Answer from the drawing. Dimensions are ordinates in mm from the lowest x, y and z of the part. A direction names the side the tool comes from. Give positions to 0.01 mm unless a question says otherwise; leave off trailing zeros. Order: outer loops, then holes, each group sorted by start corner. A loop starts at its lowest first (then second) coordinate and runs counter-clockwise, first axis right, second up. Notation, with made-up numbers: (-39, 30.5) - (-3, 30.5) arc R13 cw to (-3, 51.5) - close; hole circle Ø9 at (20.5, -10). An arc over 180 degrees is marked (long way). Use a Markdown table: item, result. Add a question column.
1) Find section D-D, the plane x = 18.25. Determine the outline of the cut face in (y, z).
2) Find section A-A, the plane x = 4. Determine the outline of the cut face in (y, z).
3) Find section C-C, the plane y = 3.5. Determine the outline of the cut face in (x, z), plus the area to 3 significant figures.
4) Find section B-B, the plane z = 10.5. Determine the outline of the cut face in (x, y).
5) Flat-ended cylindrical pins translate along their axes: pin 1 (6 mm diameter, centred on x = 12, z = 7.5, fed in from +Y); pin 2 (1.5 mm diameter, centred on x = 4, y = 4, fed in from +Z); pin 3 (1.5 mm diameter, centred on x = 4, z = 6, fed in from +Y). Find the tip coordinate at first contact, or state that the pin passes through.
6) For the marked faces 1 and 2, determine the directions among +Z, -Z, +X, -X, +Y, -Y from which every point of the face is accessible in a straight line to the end or side of a thin tool.
7) Straight lines are drawn through the part: line 1 (X direction, y = 0.5, z = 10.5); line 2 (Y direction, x = 2.15, z = 3); line 3 (X direction, y = 1.2, z = 4.5). For each, find the intervals that lie inside material, in ascending order.
8) The mould has two halves that part along X. Classify the marked faces 3, 4, 5 and 6: released by +X, released by -X, zero draft, split by the parting line, or undercut.
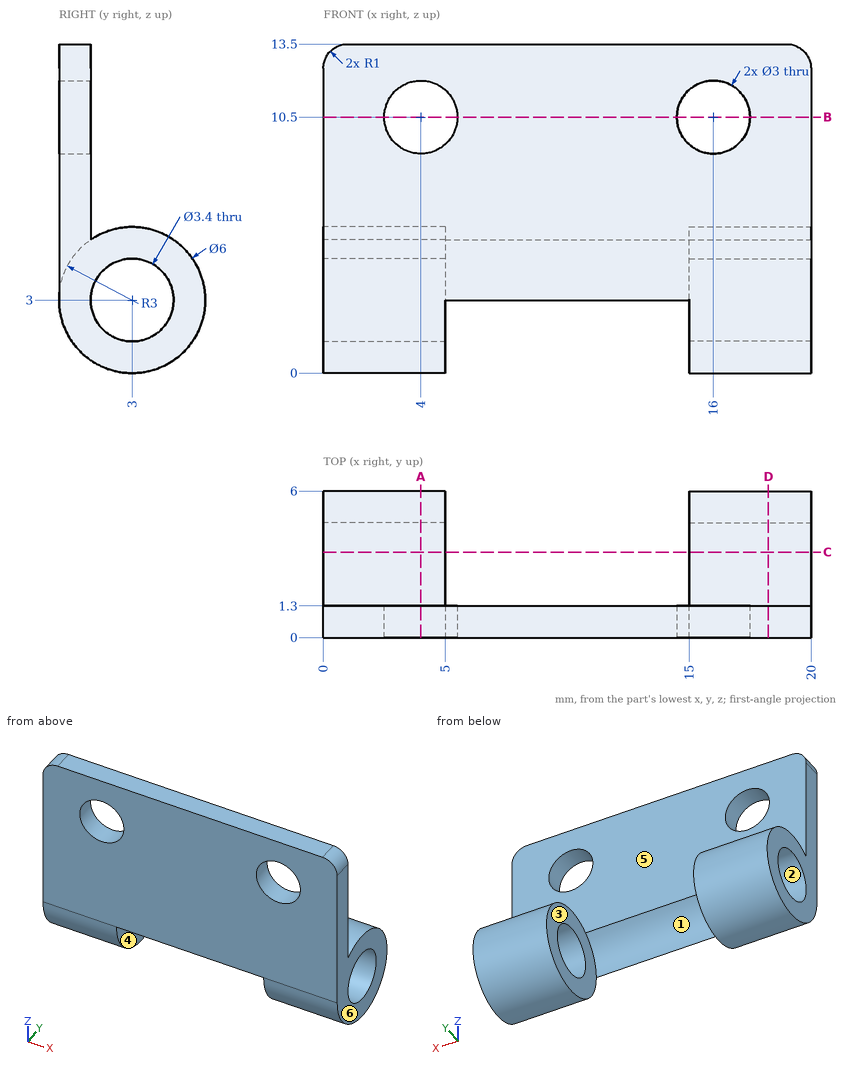
The answers:
| question | item | result |
|---|---|---|
| 1 | outline | (0, 3) arc R3 ccw (long way) to (1.3, 5.47) - (1.3, 13.5) - (0, 13.5) - close; hole circle Ø3.4 at (3, 3) |
| 2 | outline | (0, 3) arc R3 ccw (long way) to (1.3, 5.47) - (1.3, 9) - (0, 9) - close; (0, 12) - (1.3, 12) - (1.3, 13.5) - (0, 13.5) - close; hole circle Ø3.4 at (3, 3) |
| 3 | outline | (0, 0.04) - (5, 0.04) - (5, 1.38) - (0, 1.38) - close; (0, 4.62) - (5, 4.62) - (5, 5.96) - (0, 5.96) - close; (15, 0.04) - (20, 0.04) - (20, 1.38) - (15, 1.38) - close; (15, 4.62) - (20, 4.62) - (20, 5.96) - (15, 5.96) - close |
| 3 | area | 26.7 mm2 |
| 4 | outline | (0, 0) - (2.5, 0) - (2.5, 1.3) - (0, 1.3) - close; (5.5, 0) - (14.5, 0) - (14.5, 1.3) - (5.5, 1.3) - close; (17.5, 0) - (20, 0) - (20, 1.3) - (17.5, 1.3) - close |
| 5 | pin 1 | y = 1.3 |
| 5 | pin 2 | z = 5.99 |
| 5 | pin 3 | y = 4.98 |
| 6 | face 1 | -Z, +Y |
| 6 | face 2 | +X, -X |
| 7 | line 1 | 0 to 2.5, 5.5 to 14.5, 17.5 to 20 |
| 7 | line 2 | 0 to 1.3, 4.7 to 6 |
| 7 | line 3 | 0 to 5, 15 to 20 |
| 8 | face 3 | undercut |
| 8 | face 4 | undercut |
| 8 | face 5 | zero draft |
| 8 | face 6 | released by +X |
